Geometry: see drawing. Coordinates: mm, zero at the bounding-box minimum. A direction names the side the tool comes from. Give positions to 0.01 mm unless a question says otherwise; leave off trailing zeros. Loops run counter-clockwise (first coordinate to the right, second up) from the corner with the lowest first, then second, coordinate; pieces in that order, holes last. Notation, with made-up numbers: M 36.25,89.25 L 90.25,89.25 A5 ccw 90.25,95.25 Z; hole C -32,67 d2. An arc over 180 degrees is marked long. Use a Markdown table: item, result. Add a question column.
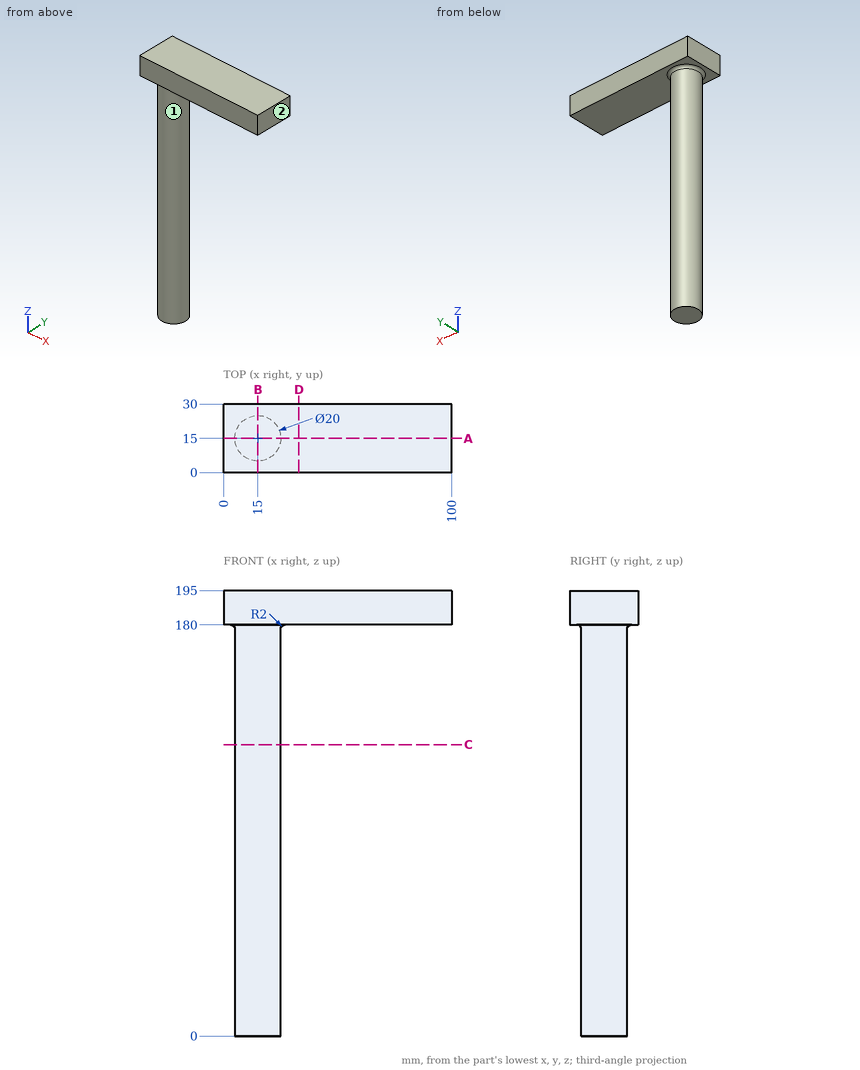
1) Section query D-D, the plane x = 33. Return the cut outline in (y, z).
2) Reachability of the marked faces 1 and 2 from +Z, -Z, +X, -X, +Y, -Y: full face, straight path, thin tool, end or side. Return the list, or none.
3) Section query B-B, the plane x = 15. Return the cut outline in (y, z), and give its area (3 significant figures).
4) Ray query, line 1 (Z direction, x = 58, y = 26.25); line 2 (Y direction, x = 14.5, z = 68.5); line 3 (Y direction, x = 16, z = 161.5). Return the intervals inside material, ascending. Write a range as [from, to].
5) Section query A-A, the plane y = 15. Return the cut outline in (x, z), and give its area (3 significant figures).
6) Section query C-C, the plane z = 127.5. Return the cut outline in (x, y), and give its area (3 significant figures).
7) Contact query for flat-ended pins moving along their axis: P1, Ø5, axis at y = 16, z = 86, coming from the -X side; P2, Ø3, axis at y = 12, z = 33, coming from the +X side; P3, Ø5, axis at x = 64.5, y = 21, coming from the -Z side. Output: stop coordinate, or through.
Entries:
| question | item | result |
|---|---|---|
| 1 | outline | M 0,180 L 30,180 L 30,195 L 0,195 Z |
| 2 | face 1 | -Z |
| 2 | face 2 | +Z, -Z, +X, +Y, -Y |
| 3 | outline | M 0,180 L 3,180 A2 cw 5,178 L 5,0 L 25,0 L 25,178 A2 cw 27,180 L 30,180 L 30,195 L 0,195 Z |
| 3 | area | 4,050 mm² |
| 4 | line 1 | z = [180, 195] |
| 4 | line 2 | y = [5.01, 24.99] |
| 4 | line 3 | y = [5.05, 24.95] |
| 5 | outline | M 0,180 L 3,180 A2 cw 5,178 L 5,0 L 25,0 L 25,178 A2 cw 27,180 L 100,180 L 100,195 L 0,195 Z |
| 5 | area | 5,100 mm² |
| 6 | outline | C 15,15 d20 |
| 6 | area | 314 mm² |
| 7 | P1 | stops at x = 5 |
| 7 | P2 | stops at x = 24.89 |
| 7 | P3 | stops at z = 180 |
